```python
from build123d import *

# Parameters (mm, degrees)
MAIN_DEPTH         = 25
SKETCH2_R          = 5.15
ROLLINGHOLE_DEPTH  = 5
SKETCH3_R          = 4
CUT_EXTRUDE2_DEPTH = 8
SKETCH4_R          = 1.6
FIXHOLE_DEPTH      = 13
SKETCH5_W          = 10
SKETCH5_H          = 6
CUT_EXTRUDE4_DEPTH = 16


with BuildPart() as part:
    # Sketch1 → Main (new body)
    with BuildSketch(Plane.XY):
        Polygon((-5.1, 0), (-5.1, -3), (-7.5, -3), (-7.5, 9), (7.5, 9), (7.5, -3), (5.1, -3), (5.1, 0), (1.45, 0), (1.45, -1), (-1.45, -1), (-1.45, 0), align=None)
    extrude(amount=MAIN_DEPTH)

    # Sketch2 → RollingHole (cut)
    with BuildSketch(Plane(origin=(0, 9, 0), x_dir=(1, 0, 0), z_dir=(0, 1, 0))):
        with Locations((0, -17.5)):
            Circle(SKETCH2_R)
    extrude(amount=-ROLLINGHOLE_DEPTH, mode=Mode.SUBTRACT)

    # Sketch3 → Cut-Extrude2 (cut, through all)
    with BuildSketch(Plane(origin=(0, 4, 0), x_dir=(1, 0, 0), z_dir=(0, 1, 0))):
        with Locations((0, -17.5)):
            Circle(SKETCH3_R)
    extrude(amount=-CUT_EXTRUDE2_DEPTH, mode=Mode.SUBTRACT)

    # Sketch4 → FixHole (cut, through all)
    with BuildSketch(Plane(origin=(0, 9, 0), x_dir=(1, 0, 0), z_dir=(0, 1, 0))):
        with Locations((0, -5)):
            Circle(SKETCH4_R)
    extrude(amount=-FIXHOLE_DEPTH, mode=Mode.SUBTRACT)

    # Sketch5 → Cut-Extrude4 (cut, through all)
    with BuildSketch(Plane.ZY.offset(7.5)):
        with Locations((5, 6)):
            Rectangle(SKETCH5_W, SKETCH5_H)
    extrude(amount=-CUT_EXTRUDE4_DEPTH, mode=Mode.SUBTRACT)


solid = part.part
```
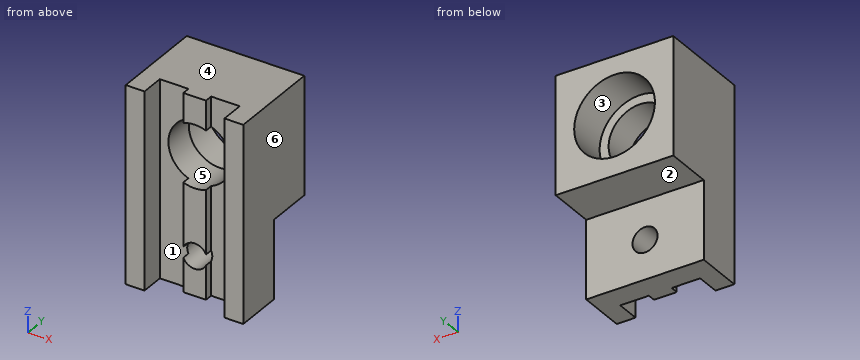
Work out the finished part from the listing and answer in its coordinate system (mm). Face numbers are marked on the shaded views. A direction names the side the tool comes from. Round coordinates to 2 decimals unless told otherwise and drop trailing zeros. Order: outer loops, then holes, each group sorted by start corner. A loop starts at its lowest first (then second) coordinate and runs counter-clockwise, first axis right, second up.
Q1. A cutting plane is placed at D-D, the plane z = 23.75. Determine the outline of the cut face in (x, y), then the cut area to 3 significant figures.
Solution:
outline: (-7.5, -3) - (-5.1, -3) - (-5.1, 0) - (-1.45, 0) - (-1.45, -1) - (1.45, -1) - (1.45, 0) - (5.1, 0) - (5.1, -3) - (7.5, -3) - (7.5, 9) - (-7.5, 9) - close
area: 152 mm2
Q2. A cutting plane is placed at A-A, the plane x = 0. Determine the outline of the cut face in (y, z).
Solution:
outline: (-1, 0) - (3, 0) - (3, 3.4) - (-1, 3.4) - close; (-1, 6.6) - (3, 6.6) - (3, 10) - (9, 10) - (9, 12.35) - (4, 12.35) - (4, 13.5) - (-1, 13.5) - close; (-1, 21.5) - (4, 21.5) - (4, 22.65) - (9, 22.65) - (9, 25) - (-1, 25) - close
Q3. A cutting plane is placed at C-C, the plane y = 7.5. Determine the outline of the cut face in (x, z), then the cut area to 3 significant figures.
Solution:
outline: (-7.5, 10) - (7.5, 10) - (7.5, 25) - (-7.5, 25) - close; hole circle Ø10.3 at (0, 17.5)
area: 142 mm2
Q4. The mould has two halves that part along X. Classify the marked faces 4, 5 and 6: pulls with the +X half, pulls with the -X half, needs draft (parallel to the pull), parting line crosses it, or undercut.
Solution:
face 4: needs draft
face 5: undercut
face 6: pulls with the +X half
Q5. Find the intervals of material crossed by line 1 along Z through (x, y) = (0, 2.8); line 2 along X through (y, z) = (5.4, 17.5); line 3 along Z through (x, y) = (1, 2.5), in increasing order.
Solution:
line 1: z = 0 to 3.4, 6.6 to 13.5, 21.5 to 25
line 2: x = -7.5 to -5.15, 5.15 to 7.5
line 3: z = 0 to 3.75, 6.25 to 13.63, 21.37 to 25
Q6. A cutting plane is placed at B-B, the plane z = 5. Determine the outline of the cut face in (x, y).
Solution:
outline: (-7.5, -3) - (-5.1, -3) - (-5.1, 0) - (-1.6, 0) - (-1.6, 3) - (-7.5, 3) - close; (1.6, 0) - (5.1, 0) - (5.1, -3) - (7.5, -3) - (7.5, 3) - (1.6, 3) - close
Q7. A tool of negligible diameter and unlimited length cuts with its end or side. For the marked faces 1, 2 and 3, from which of +Z, -Z, +X, -X, +Y, -Y can it reach the whole face along a straight path? Write none if from no direction.
Solution:
face 1: +Z, -Z, -Y
face 2: -Z, +X, -X, +Y
face 3: +Y
Q8. Given pin 1 Ø3.5 at (x, z) = (0, 5) entering from -Y; pin 2 Ø5 at (x, z) = (0, 20) entering from +Y; pin 3 Ø3 at (x, z) = (-3.5, 3.5) entering from +Y, each flat-ended and moving along its own axis, determine where each tip first touches the part or whether it passes through.
Solution:
pin 1: stops at y = -1
pin 2: stops at y = 4
pin 3: stops at y = 3
